```python
from build123d import *

# Parameters (mm, degrees)
SKETCH1_W           = 10.253048328
SKETCH1_H           = 10.253048328
BOSS_EXTRUDE1_DEPTH = 13.5
SKETCH2_R           = 0.65
BOSS_EXTRUDE2_DEPTH = 1
FILLET3_R           = 0.3


with BuildPart() as part:
    # Sketch1 → Boss-Extrude1 (new body)
    with BuildSketch(Plane(origin=(0, 0, 0), x_dir=(1, 0, 0), z_dir=(0, 1, 0))):
        Rectangle(SKETCH1_W, SKETCH1_H)
    extrude(amount=BOSS_EXTRUDE1_DEPTH)

    # Sketch2 → Boss-Extrude2 (add)
    with BuildSketch(Plane(origin=(0, 13.5, 0), x_dir=(1, 0, 0), z_dir=(0, 1, 0))):
        with Locations(Location((0, 0, 0), (0, 0, 90))):  # turned: the seam where the file's is
            Circle(SKETCH2_R)
    extrude(amount=BOSS_EXTRUDE2_DEPTH)

    # Fillet3
    fillet3_edges = [part.edges().sort_by_distance(p)[0] for p in [
        (-5.126524164, 13.5, 0),
        (0, 13.5, 0.65),
        (0, 13.5, 5.126524164),
        (5.126524164, 13.5, 0),
        (5.126524164, 6.75, 5.126524164),
        (-5.126524164, 6.75, 5.126524164),
        (-5.126524164, 6.75, -5.126524164),
        (5.126524164, 6.75, -5.126524164),
        (0, 13.5, -5.126524164),
    ]]
    fillet(fillet3_edges, radius=FILLET3_R)


solid = part.part
```
Read the model definition and answer for the solid it produces. Units are mm, in the model's axes. A direction names the side the tool comes from. Coordinates: 2 decimals unless noted, no trailing zeros. Loops run counter-clockwise (first coordinate to the right, second up) from the corner with the lowest first, then second, coordinate; pieces in that order, holes last. Notation, with made-up numbers: (-9, -19.75) - (32, -19.75) arc R12 ccw to (32, -11.75) - close; hole circle Ø10 at (43, 36.25). An arc over 180 degrees is marked (long way). Answer in a Markdown table with one row per item.
1. Find section A-A, the plane x = 4.25. Write down the section's boundary in (y, z).
Conclusion:
| item | result |
|---|---|
| outline | (0, -5.13) - (13.2, -5.13) arc R0.3 ccw to (13.5, -4.83) - (13.5, 4.83) arc R0.3 ccw to (13.2, 5.13) - (0, 5.13) - close |
2. Find section D-D, the plane z = 0. Write down the section's boundary in (x, y), then the cut area to 3 significant figures.
Conclusion:
| item | result |
|---|---|
| outline | (-5.13, 0) - (5.13, 0) - (5.13, 13.2) arc R0.3 ccw to (4.83, 13.5) - (0.95, 13.5) arc R0.3 cw to (0.65, 13.8) - (0.65, 14.5) - (-0.65, 14.5) - (-0.65, 13.8) arc R0.3 cw to (-0.95, 13.5) - (-4.83, 13.5) arc R0.3 ccw to (-5.13, 13.2) - close |
| area | 140 mm² |
3. Find section C-C, the plane x = 0. Write down the section's boundary in (y, z), then the cut area to 3 significant figures.
Conclusion:
| item | result |
|---|---|
| outline | (0, -5.13) - (13.2, -5.13) arc R0.3 ccw to (13.5, -4.83) - (13.5, -0.95) arc R0.3 cw to (13.8, -0.65) - (14.5, -0.65) - (14.5, 0.65) - (13.8, 0.65) arc R0.3 cw to (13.5, 0.95) - (13.5, 4.83) arc R0.3 ccw to (13.2, 5.13) - (0, 5.13) - close |
| area | 140 mm² |
4. A straight line is drawn through the part: line 1 (Y direction, x = -1.5, z = -1.75). Find the intervals that lie inside material, in ascending order.
Conclusion:
| item | result |
|---|---|
| line 1 | y = 0 to 13.5 |
5. Find section B-B, the plane z = 2.25. Write down the section's boundary in (x, y).
Conclusion:
| item | result |
|---|---|
| outline | (-5.13, 0) - (5.13, 0) - (5.13, 13.2) arc R0.3 ccw to (4.83, 13.5) - (-4.83, 13.5) arc R0.3 ccw to (-5.13, 13.2) - close |
6. Which of the six approach directions +Z, -Z, +X, -X, +Y, -Y give full straight-line access (tool end or side, diameter ignored) to faces 4 (the face through (-0.2, 14.15, -0.62)), 5 (the face through (0, 7, -5.127))?
Conclusion:
| item | result |
|---|---|
| face 4 | +Y |
| face 5 | -Z, +X, -X, +Y, -Y |
7. Determine the mould class of faces 1 (the face through (0, 0, 0)), 2 (the face through (0, 7, 5.127)), 3 (the face through (-1.1, 13.5, -0.1)) for opening direction Y: +Y half, -Y half, draft (parallel to the pull), parting line (faces both ways), or undercut.
Conclusion:
| item | result |
|---|---|
| face 1 | -Y half |
| face 2 | draft |
| face 3 | +Y half |
